from build123d import *

# Parameters (mm, degrees)
SKETCH1_R            = 50.8
BOSS_EXTRUDE1_DEPTH  = 38.1
CUT_EXTRUDE1_REACH   = 83.32
SKETCH2_W            = 43.18
SKETCH2_H            = 44.45
FILLET1_R            = 6.35
M3_CLEARANCE_HOLE1_D = 3.4


with BuildPart() as part:
    # Sketch1 → Boss-Extrude1 (new body)
    with BuildSketch(Plane(origin=(0, 0, 0), x_dir=(1, 0, 0), z_dir=(0, 1, 0))):
        with Locations(Location((0, 0, 0), (0, 0, 90))):
            Circle(SKETCH1_R)
    extrude(amount=BOSS_EXTRUDE1_DEPTH)

    # Sketch2 → Cut-Extrude1 (cut, up to next)
    with BuildSketch(Plane(origin=(0, 38.1, 0), x_dir=(1, 0, 0), z_dir=(0, 1, 0)), mode=Mode.PRIVATE) as cut_extrude1_sk1:
        with Locations((0, -28.575)):
            Rectangle(SKETCH2_W, SKETCH2_H)
    cut_extrude1_tool1 = extrude(cut_extrude1_sk1.sketch, amount=-CUT_EXTRUDE1_REACH, mode=Mode.PRIVATE) & part.part
    add(cut_extrude1_tool1.solids().sort_by_distance((0, 38.1, 28.575))[0], mode=Mode.SUBTRACT)

    # Fillet1
    fillet1_edges = [part.edges().sort_by_distance(p)[0] for p in [
        (-21.59, 19.05, 6.35),
        (21.59, 19.05, 6.35),
    ]]
    fillet(fillet1_edges, radius=FILLET1_R)

    # M3 Clearance Hole1 (through all)
    with Locations(Plane(origin=(0, 38.1, 0), x_dir=(1, 0, 0), z_dir=(0, 1, 0))):
        with Locations((0, 0)):
            Hole(M3_CLEARANCE_HOLE1_D / 2)


solid = part.part
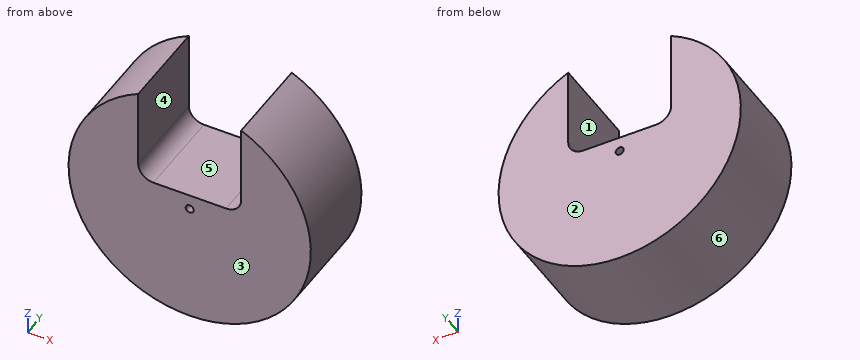
Here's how the part is built. I have some questions about the finished solid (model axes, mm). Face numbers are marked on the shaded views. A direction names the side the tool comes from. Round coordinates to 2 decimals unless told otherwise and drop trailing zeros. Loops run counter-clockwise (first coordinate to the right, second up) from the corner with the lowest first, then second, coordinate; pieces in that order, holes last. Notation, with made-up numbers: M 43.25,48.5 L 95.25,48.5 A21 cw 95.25,75.5 Z; hole C -24.75,38.25 d3. An arc over 180 degrees is marked long. Write each question's results on one line, items separated by ' | '. Start each with the question number.
(1) On a 3-axis mill with a long thin cutter (end or side, diameter ignored), from which of +Z, -Z, +X, -X, +Y, -Y can I reach the whole of each face in a straight line? I mean the marked faces 1 and 2. Say none if no direction works.
(2) I want a section at C-C (y = 33.5). Please give me the cut outline in (x, z).
(3) If I drill on probe 1 along Z at (x, y) = (0, 12); probe 2 along X at (y, z) = (27.5, 27); probe 3 along X at (y, z) = (20, 20.5), over which ranges is the centre line in solid material (lowest first)? Write a range as from..to.
(4) I want a section at B-B (x = 0). Please give me the cut outline in (y, z).
(5) Thinking about a two-plate mould opening in X: for the marked faces 3, 4, 5 and 6, which applies, pulls with the +X half, pulls with the -X half, needs draft (parallel to the pull), parting line crosses it, or undercut?
(6) I want a section at D-D (x = 12.5). Please give me the cut outline in (y, z), then the cut area to 3 significant figures.
(7) I want a section at A-A (z = 20.5). Please give me the cut outline in (x, y).
(8) Will these pins go through, and if not, where does the flat tip stop? P1, Ø16.5, axis at y = 11.5, z = 30.5, coming from the +X side; P2, Ø3, axis at y = 5, z = 33, coming from the -X side; P3, Ø10, axis at y = 24.5, z = 34.5, coming from the -X side; P4, Ø3, axis at x = 0, z = 0, coming from the +Y side.
Solved:
1) face 1: +Z, +Y, -Y | face 2: +Z, -Z, +X, -X, +Y
2) outline: M -21.59,12.7 L -21.59,45.98 A50.8 ccw long 21.59,45.98 L 21.59,12.7 A6.35 cw 15.24,6.35 L -15.24,6.35 A6.35 cw Z; hole C 0,0 d3.4
3) probe 1: z = -50.8..-1.7, 1.7..6.35 | probe 2: x = -43.03..-21.59, 21.59..43.03 | probe 3: x = -46.48..-21.59, 21.59..46.48
4) outline: M 0,-50.8 L 38.1,-50.8 L 38.1,-1.7 L 0,-1.7 Z; M 0,1.7 L 38.1,1.7 L 38.1,6.35 L 0,6.35 Z
5) face 3: needs draft | face 4: undercut | face 5: undercut | face 6: parting line crosses it
6) outline: M 0,-49.24 L 38.1,-49.24 L 38.1,6.35 L 0,6.35 Z | area: 2,120 mm²
7) outline: M -46.48,0 L -21.59,0 L -21.59,38.1 L -46.48,38.1 Z; M 21.59,0 L 46.48,0 L 46.48,38.1 L 21.59,38.1 Z
8) P1: stops at x = 45.67 | P2: stops at x = -39.85 | P3: stops at x = -41.36 | P4: passes through
